The listing builds one solid part. Answer for the finished solid, in the listing's coordinates (mm). A direction names the side the tool comes from. Give positions to 0.01 mm unless a question says otherwise; leave off trailing zeros. Loops run counter-clockwise (first coordinate to the right, second up) from the corner with the lowest first, then second, coordinate; pieces in that order, holes last.
Item 1: Consider line 1 along X through (y, z) = (-2.8, 14); line 2 along X through (y, z) = (-1.45, 13); line 3 along X through (y, z) = (-1.2, -16). Determine where each line is inside the solid, lowest interval first.
Item 2: The mould has two halves that part along X. Classify faces 3 (the face through (188.87, -1.48, 20.98)), 4 (the face through (-135.854, -1.521, 15.489)), 5 (the face through (163.539, -1.479, -3.924)): pulls with the +X half, pulls with the -X half, needs draft (parallel to the pull), parting line crosses it, or undercut.
Item 3: Each of these flat-tipped pins is pushed along its axis until it touches: pin 1 Ø1.5 at (x, y) = (49.5, -2) entering from -Z; pin 2 Ø1.5 at (y, z) = (-1, -19.5) entering from -X. Where does it stop, or does it pass through?
Item 4: Section B-B, the plane x = -33.5 is taken. Give the vertices of the cut face in (y, z), and give its area (3 significant figures).
Item 5: A tool of negligible diameter and unlimited length cuts with its end or side. For faces 1 (the face through (-107.07, -1.48, 9.24)), 2 (the face through (-98.02, -1.48, -4.03)), from which of +Z, -Z, +X, -X, +Y, -Y can it reach the whole face along a straight path? Write none if from no direction.
Item 6: Section A-A, the plane y = -1.3 is taken. Give the number of separate pieces and of enclosed holes in the cut face, and give its area (3 significant figures).
from build123d import *

# Parameters (mm, degrees)
F0_R     = 2.25
F0_R_2   = 5.5
F0_R_3   = 2.75
F1_DEPTH = 3
F2_R     = 6
F3_R     = 15


# Not quite as in the source:
# - ends of sketch curves that miss each other by under 0.0002 mm in the source are joined


with BuildPart() as f1:
    # F0 (on Front) → F1 (new body)
    with BuildSketch(Plane.XZ):
        with BuildLine():
            Line((167.4230358146, 30.0005254045), (-101.5769641849, 30.0000224371))
            ThreePointArc((-101.5769641849, 30.0000224371), (-122.790151189, 21.2131862095), (-131.576908088, -3.36535e-05))
            Line((-131.576908088, -3.36535e-05), (-131.5768594728, -26.0000336567))
            Line((-131.5768594728, -26.0000336567), (-113.5768594728, -26))
            Line((-113.5768594728, -26), (-113.5768594728, -18))
            Line((-113.5768594728, -18), (-113.57685947, -9))
            Line((-113.57685947, -9), (-113.5768594672, 0))
            Line((-113.5768594672, 0), (-85.4137075401, 0))
            Line((-85.4137075401, 0), (149.4231405226, 0))
            Line((149.4231405226, 0), (151.260137769, 0))
            Line((151.260137769, 0), (179.4231405277, -8.9999831717))
            Line((179.4231405277, -8.9999831717), (179.4231405277, -17.9999663433))
            Line((179.4231405277, -17.9999663433), (179.4231405277, -26))
            Line((179.4231405277, -26), (197.4231405276, -25.9999663433))
            Line((197.4231405276, -25.9999663433), (197.4230919114, 0.0005814952))
            ThreePointArc((197.4230919114, 0.0005814952), (188.6362556816, 21.2137685033), (167.4230358146, 30.0005254045))
        make_face()
        with Locations((-126.5768744313, -18.0000243076)):
            Circle(F0_R, mode=Mode.SUBTRACT)
        with Locations((-118.5768744313, -18.0000093491)):
            Circle(F0_R, mode=Mode.SUBTRACT)
        with Locations((184.4231255691, -17.9999663433)):
            Circle(F0_R, mode=Mode.SUBTRACT)
        with Locations((192.4231255691, -17.9999663442)):
            Circle(F0_R, mode=Mode.SUBTRACT)
        with Locations((-120.0769249193, 8.9998906191)):
            Circle(F0_R, mode=Mode.SUBTRACT)
        with Locations((-101.5769249198, 9.0000224409)):
            Circle(F0_R_2, mode=Mode.SUBTRACT)
        with Locations((-83.0769249199, 8.9999598022)):
            Circle(F0_R, mode=Mode.SUBTRACT)
        with Locations((148.9230750802, 9.0003935993)):
            Circle(F0_R, mode=Mode.SUBTRACT)
        with Locations((167.4230750797, 9.0005254008)):
            Circle(F0_R_2, mode=Mode.SUBTRACT)
        with Locations((185.9230750796, 9.0004627825)):
            Circle(F0_R, mode=Mode.SUBTRACT)
        with BuildLine():
            ThreePointArc((-131.576908088, -3.36535e-05), (-122.790151189, 21.2131862095), (-101.5769641849, 30.0000224371))
            Line((-101.5769641849, 30.0000224371), (-146.5769641849, 29.999966344))
            Line((-146.5769641849, 29.999966344), (-146.5769517198, 19.999966344))
            Line((-146.5769517198, 19.999966344), (-131.576908088, 19.999966344))
            Line((-131.576908088, 19.999966344), (-131.576908088, -3.36535e-05))
        make_face()
        with Locations((-140.5769579523, 24.999966344)):
            Circle(F0_R_3, mode=Mode.SUBTRACT)
        with Locations((-129.5769910358, 25.0335049432)):
            Circle(F0_R_3, mode=Mode.SUBTRACT)
        Polygon((-113.5768594672, 0), (-113.57685947, -9), (-85.4137075401, 0), align=None)
    extrude(amount=F1_DEPTH)

    # F2
    f2_edges = [f1.edges().sort_by_distance(p)[0] for p in [
        (-113.576859, -1.5, -9),
        (-85.413708, -1.5, 0),
        (151.260138, -1.5, 0),
        (179.423141, -1.5, -8.999983),
    ]]
    fillet(f2_edges, radius=F2_R)

    # F3
    f3_edges = [f1.edges().sort_by_distance(p)[0] for p in [
        (-131.576908, -1.5, 19.999966),
    ]]
    fillet(f3_edges, radius=F3_R)


solid = f1.part
Worked answers:
1. line 1: x = -134.58 to -103.87, -99.29 to 165.13, 169.72 to 193.96
1. line 2: x = -133.89 to -105.35, -97.8 to 163.65, 171.2 to 194.46
1. line 3: x = -131.58 to -127.61, -125.55 to -119.61, -117.55 to -113.58, 179.42 to 183.39, 185.45 to 191.39, 193.45 to 197.42
2. face 3: pulls with the +X half
2. face 4: pulls with the -X half
2. face 5: undercut
3. pin 1: stops at z = 0
3. pin 2: stops at x = -131.58
4. outline: (-3, 0) - (0, 0) - (0, 30) - (-3, 30) - close
4. area: 90.0 mm2
5. face 1: +Y, -Y
5. face 2: -Z, +Y, -Y
6. separate pieces: 1
6. enclosed holes: 12
6. area: 10,700 mm2
